from build123d import *

# Parameters (mm, degrees)
SKETCH1_R               = 38.05
SKETCH1_R_2             = 29
BOSS_EXTRUDE1_DEPTH     = 15
SKETCH3_R               = 21.5
SKETCH3_R_2             = 18.5
SKETCH3_R_3             = 54.301992004
SKETCH3_R_4             = 51.301992004
SKETCH3_W               = 3
SKETCH3_H               = 32.801992004
CUT_EXTRUDE_THIN1_DEPTH = 7.5


with BuildPart() as part:
    # Sketch1 → Boss-Extrude1 (new body)
    with BuildSketch(Plane(origin=(0, 0, 0), x_dir=(1, 0, 0), z_dir=(0, 1, 0))):
        Circle(SKETCH1_R)
        Circle(SKETCH1_R_2, mode=Mode.SUBTRACT)
    extrude(amount=BOSS_EXTRUDE1_DEPTH)

    # Sketch3 → Cut-Extrude-Thin1 (cut)
    with BuildSketch(Plane(origin=(0, 15, 0), x_dir=(1, 0, 0), z_dir=(0, 1, 0))):
        Circle(SKETCH3_R)
        Circle(SKETCH3_R_2, mode=Mode.SUBTRACT)
        Circle(SKETCH3_R_3)
        Circle(SKETCH3_R_4, mode=Mode.SUBTRACT)
        with Locations((0, -36.400996002)):
            Rectangle(SKETCH3_W, SKETCH3_H)
        Polygon((-16.570508076, 11.299038106), (-44.977866446, 27.700034108), (-46.477866446, 25.101957897), (-18.070508076, 8.700961894), align=None)
        Polygon((18.070508076, 8.700961894), (46.477866446, 25.101957897), (44.977866446, 27.700034108), (16.570508076, 11.299038106), align=None)
    extrude(amount=-CUT_EXTRUDE_THIN1_DEPTH, mode=Mode.SUBTRACT)


solid = part.part
Here's how the part is built. I have some questions about the finished solid (model axes, mm). A direction names the side the tool comes from. Coordinates: 2 decimals unless noted, no trailing zeros. Write each loop counter-clockwise with the first axis right and the second up, starting at its lowest first coordinate (ties: lowest second). Pieces come first, ordered by that corner, then holes.
Item 1: I want a section at C-C on x = 0. Write out the boundary of the cut face in (y, z).
Item 2: If we mould it in two halves opening along Z, with no side actions, what happens to faces 4 (the flat face through (1.5, 11, 34)), 5 (the cylindrical face through (13.38, 7.4, 25.73)), 6 (the cylindrical face through (20.46, 7.4, -32.08))? For each: +Z half, -Z half, draft (parallel to the pull), parting line (faces both ways), or undercut.
Item 3: I want a section at D-D on y = 3.5. Write out the boundary of the cut face in (x, z), and give its area (3 significant figures).
Item 4: If I drill on line 1 (X direction, y = 4.5, z = 0); line 2 (Z direction, x = 0, y = 10.5), over which ranges is the centre line in solid material (lowest first)?
Item 5: Will these pins go through, and if not, where does the flat tip stop? pin 1 (5 mm diameter, centred on y = 11.5, z = 22.5, fed in from -X); pin 2 (8 mm diameter, centred on x = 6, y = 3, fed in from +Z); pin 3 (3 mm diameter, centred on y = 9, z = -19, fed in from +X).
Item 6: I want a section at A-A on z = 0. Write out the boundary of the cut face in (x, y).
Item 7: On a 3-axis mill with a long thin cutter (end or side, diameter ignored), from which of +Z, -Z, +X, -X, +Y, -Y can I reach the whole of each face in a straight line? I mean faces 1 (the flat face through (-1.5, 11, 34)), 2 (the flat face through (-9, 0, 28)), 3 (the flat face through (29.699, 11.302, -15.415)). Say none if no direction works.
Item 8: I want a section at B-B on y = 9.25. Write out the boundary of the cut face in (x, z).
Findings below:
1. outline: (0, -38.05) - (15, -38.05) - (15, -29) - (0, -29) - close; (0, 29) - (7.5, 29) - (7.5, 38.05) - (0, 38.05) - close
2. face 4: draft
2. face 5: undercut
2. face 6: parting line
3. outline: circle Ø76.1 at (0, 0); hole circle Ø58 at (0, 0)
3. area: 1,910 mm2
4. line 1: x = -38.05 to -29, 29 to 38.05
4. line 2: z = -38.05 to -29
5. pin 1: stops at x = -32.37
5. pin 2: stops at z = 38
5. pin 3: stops at x = 33.79
6. outline: (-38.05, 0) - (-29, 0) - (-29, 15) - (-38.05, 15) - close; (29, 0) - (38.05, 0) - (38.05, 15) - (29, 15) - close
7. face 1: +Z, +Y
7. face 2: +Z, -Z, +X, -X, -Y
7. face 3: +Y
8. outline: (-33.68, -17.71) - (-25.83, -13.18) arc R29 cw to (-1.5, 28.96) - (-1.5, 38.02) arc R38.05 ccw to start; (-32.18, -20.31) arc R38.05 ccw to (32.18, -20.31) - (24.33, -15.78) arc R29 cw to (-24.33, -15.78) - close; (1.5, 28.96) arc R29 cw to (25.83, -13.18) - (33.68, -17.71) arc R38.05 ccw to (1.5, 38.02) - close
